```python
from build123d import *

# Parameters (mm, degrees)
F0_W     = 43.4223142958
F0_H     = 102.4999973916
F1_DEPTH = 3
F2_D     = 12
F2_DEPTH = 50
F2_TIP   = 3.6051637142
F3_D     = 5
F3_DEPTH = 50
F3_TIP   = 1.5021515476


with BuildPart() as f1:
    # F0 (on Top) → F1 (new body)
    with BuildSketch(Plane.XY):
        Polygon((-29.4820813204, 57.3426440605), (-29.4820813204, -77.9801009848), (29.4820813204, -77.9801009848), (29.4820813204, 57.3426440605), (8.9785616139, 57.3426440605), (8.9785616139, 72.3426440605), (-11.0214383861, 72.3426440605), (-11.0214383861, 57.3426440605), align=None)
        with Locations((0, -13.1670495591)):
            Rectangle(F0_W, F0_H, mode=Mode.SUBTRACT)
    extrude(amount=F1_DEPTH)

    # F2
    with Locations(Plane(origin=(0, 0, 0), x_dir=(1, 0, 0), z_dir=(0, 0, -1))):
        with Locations((-1.0214383861, -67.6703378558)):
            Hole(F2_D / 2, depth=F2_DEPTH)
            with Locations((0, 0, -(F2_DEPTH + F2_TIP / 2))):  # 118° drill point
                Cone(0, F2_D / 2, F2_TIP, mode=Mode.SUBTRACT)

    # F3
    with Locations(Plane(origin=(0, 0, 0), x_dir=(1, 0, 0), z_dir=(0, 0, -1))):
        with Locations((0, -42.3597060144), (0, 74.8838037252)):
            Hole(F3_D / 2, depth=F3_DEPTH)
            with Locations((0, 0, -(F3_DEPTH + F3_TIP / 2))):  # 118° drill point
                Cone(0, F3_D / 2, F3_TIP, mode=Mode.SUBTRACT)


solid = f1.part
```
The model under review builds one solid part; all positions refer to its coordinate system, in mm. A direction names the side the tool comes from. Coordinates: 2 decimals unless noted, no trailing zeros. Loops run counter-clockwise (first coordinate to the right, second up) from the corner with the lowest first, then second, coordinate; pieces in that order, holes last. Notation, with made-up numbers: (65.25, 3) -> (104.25, 3) arc R32 cw to (104.25, 40) -> close; hole circle Ø7 at (45.5, 65). An arc over 180 degrees is marked (long way). Answer as CSV lines item,"result".
Item 1: Take a section at B-B, the plane x = 7.5. State the section outline as (y, z) points.
Results below:
outline,"(-77.98, 0) -> (-64.42, 0) -> (-64.42, 3) -> (-77.98, 3) -> close; (38.08, 0) -> (72.34, 0) -> (72.34, 3) -> (38.08, 3) -> close"
Item 2: Take a section at D-D, the plane x = 0.5. State the section outline as (y, z) points, and give its area (3 significant figures).
Results below:
outline,"(-77.98, 0) -> (-77.33, 0) -> (-77.33, 3) -> (-77.98, 3) -> close; (-72.43, 0) -> (-64.42, 0) -> (-64.42, 3) -> (-72.43, 3) -> close; (38.08, 0) -> (39.91, 0) -> (39.91, 3) -> (38.08, 3) -> close; (44.81, 0) -> (61.87, 0) -> (61.87, 3) -> (44.81, 3) -> close"
area,"82.6 mm2"
Item 3: Take a section at A-A, the plane y = -10. State the section outline as (x, z) points, and give its area (3 significant figures).
Results below:
outline,"(-29.48, 0) -> (-21.71, 0) -> (-21.71, 3) -> (-29.48, 3) -> close; (21.71, 0) -> (29.48, 0) -> (29.48, 3) -> (21.71, 3) -> close"
area,"46.6 mm2"
Item 4: For L1, parallel to Y at x = 0, z = 2.35; L2, parallel to X at y = 32, z = 2.8; L3, parallel to Y at x = -5, z = 1.5, list the stretches that pass through material, from the lowest coordinate up.
Results below:
L1,"y = -77.98 to -77.38, -72.38 to -64.42, 38.08 to 39.86, 44.86 to 61.76"
L2,"x = -29.48 to -21.71, 21.71 to 29.48"
L3,"y = -77.98 to -64.42, 38.08 to 63.18, 72.16 to 72.34"
Item 5: Draft analysis for pull direction X (two halves, no side actions). For faces 1 (the flat face through (8.979, 65, 1)), 2 (the flat face through (0, -77.98, 1)), 3 (the flat face through (0, 38.083, 1)), state which applies: +X half, -X half, draft (parallel to the pull), parting line (faces both ways), or undercut.
Results below:
face 1,"+X half"
face 2,"draft"
face 3,"undercut"
Item 6: Insertion check: pin 1 (1.5 mm diameter, centred on y = 64.5, z = 1, fed in from -X). The pin has a flat end and moves straight along its axis. Give the tip position at first contact, or say it passes through.
Results below:
pin 1,"stops at x = -11.02"
Item 7: Take a section at C-C, the plane z = 1.9. State the section outline as (x, y) points, and give its area (3 significant figures).
Results below:
outline,"(-29.48, -77.98) -> (29.48, -77.98) -> (29.48, 57.34) -> (8.98, 57.34) -> (8.98, 72.34) -> (2.74, 72.34) arc R6 cw (long way) to (-4.79, 72.34) -> (-11.02, 72.34) -> (-11.02, 57.34) -> (-29.48, 57.34) -> close; hole (-21.71, -64.42) -> (21.71, -64.42) -> (21.71, 38.08) -> (-21.71, 38.08) -> close; hole circle Ø5 at (0, -74.88); hole circle Ø5 at (0, 42.36)"
area,"3,680 mm2"
Item 8: Machinability: for faces 4 (the flat face through (29.482, -11, 1)), 5 (the flat face through (-21.711, -14, 1)), 6 (the flat face through (6, 72.343, 1)), 7 (the flat face through (-11.021, 65, 1)), 8 (the flat face through (19, 57.343, 1)), which of the approach directions +Z, -Z, +X, -X, +Y, -Y give a long, thin tool a straight path to every point of the face, cutting with its end or side? Answer none if there is none.
Results below:
face 4,"+Z, -Z, +X, +Y, -Y"
face 5,"+Z, -Z"
face 6,"+Z, -Z, +X, -X, +Y"
face 7,"+Z, -Z, -X, +Y"
face 8,"+Z, -Z, +X, +Y"
